from build123d import *

# Parameters (mm, degrees)
BOSS_EXTRUDE4_DEPTH = 3
SKETCH2_W           = 13.411682353
SKETCH2_H           = 48.538644398
BOSS_EXTRUDE5_DEPTH = 10


with BuildPart() as part:
    # Sketch1 → Boss-Extrude4 (new body)
    with BuildSketch(Plane.XY):
        with BuildLine():
            Line((10.190210498, 139.492737182), (-3.221471855, 139.492737182))
            ThreePointArc((-3.221471855, 139.492737182), (-21.694357927, 115.223414983), (-3.221471855, 90.954092784))
            Line((-3.221471855, 90.954092784), (10.190210498, 90.954092784))
            ThreePointArc((10.190210498, 90.954092784), (28.663096571, 115.223414983), (10.190210498, 139.492737182))
        make_face()
    extrude(amount=BOSS_EXTRUDE4_DEPTH)

    # Sketch2 → Boss-Extrude5 (add)
    with BuildSketch(Plane.XY.offset(3)):
        with Locations((3.484369322, 115.223414983)):
            Rectangle(SKETCH2_W, SKETCH2_H)
    extrude(amount=BOSS_EXTRUDE5_DEPTH)


solid = part.part
For this review, take the finished solid that the model builds, in its own axes (mm). A direction names the side the tool comes from. Give positions to 0.01 mm unless a question says otherwise; leave off trailing zeros. Order: outer loops, then holes, each group sorted by start corner. A loop starts at its lowest first (then second) coordinate and runs counter-clockwise, first axis right, second up. Notation, with made-up numbers: (62, 7.25) -> (105, 7.25) arc R29 cw to (105, 37.25) -> close; hole circle Ø3 at (6.25, 41). An arc over 180 degrees is marked (long way). Write item = value, one per line.
1) We need section C-C, the plane x = -10.5. Give the boundary of the cut face in (y, z), and give its area (3 significant figures).
Findings:
outline = (94.29, 0) -> (136.16, 0) -> (136.16, 3) -> (94.29, 3) -> close
area = 126 mm^2
2) We need section D-D, the plane y = 126.5. Give the boundary of the cut face in (x, z), and give its area (3 significant figures).
Findings:
outline = (-19.03, 0) -> (26, 0) -> (26, 3) -> (10.19, 3) -> (10.19, 13) -> (-3.22, 13) -> (-3.22, 3) -> (-19.03, 3) -> close
area = 269 mm^2
3) We need section B-B, the plane z = 1. Give the boundary of the cut face in (x, y), and give its area (3 significant figures).
Findings:
outline = (-3.22, 90.95) -> (10.19, 90.95) arc R25.18 ccw to (10.19, 139.49) -> (-3.22, 139.49) arc R25.18 ccw to start
area = 1,980 mm^2
4) Insertion check: pin 1 (3 mm diameter, centred on y = 114, z = 5.5, fed in from -X); pin 2 (3 mm diameter, centred on x = 23.5, z = 3.5, fed in from -Y); pin 3 (3 mm diameter, centred on y = 112.5, z = 5.5, fed in from +X). Each pin has a flat end and moves straight along its axis. Give the tip position at first contact, or say it passes through.
Findings:
pin_1 = -3.22
pin_2 = 98.25
pin_3 = 10.19
5) We need section A-A, the plane y = 114. Give the boundary of the cut face in (x, z), and give its area (3 significant figures).
Findings:
outline = (-21.66, 0) -> (28.63, 0) -> (28.63, 3) -> (10.19, 3) -> (10.19, 13) -> (-3.22, 13) -> (-3.22, 3) -> (-21.66, 3) -> close
area = 285 mm^2
6) To check wall thickness, follow L1, parallel to Z at x = -8.5, y = 131.5; L2, parallel to X at y = 93.5, z = 7; L3, parallel to Y at x = 26, z = 2. State the ranges of each line that lie inside material, in increasing order. Write a range as from..to.
Findings:
L1 = 0..3
L2 = -3.22..10.19
L3 = 103.95..126.49
7) For faces 1 (the face through (-3.221, 115, 8)), 2 (the face through (10.19, 115, 8)), 3 (the face through (28.66, 114.76, 1.48)), list the 3-axis set-ups (+Z, -Z, +X, -X, +Y, -Y) from which the entire face can be reached by the end or side of a thin tool; tool diameter is ignored.
Findings:
face_1 = +Z, -X, +Y, -Y
face_2 = +Z, +X, +Y, -Y
face_3 = +Z, -Z, +X
